from build123d import *

# Parameters (mm, degrees)
F1_DEPTH     = 10
F3_DEPTH     = 22
F4_DEPTH     = 48
F6_D         = 16
F6_DEPTH     = 54
F6_TIP       = 4.8068849522
F7_T1_DEPTH  = 14
F7_T4_ANGLE  = 180
F7_T5_DEPTH  = 46
F7_T7_DEPTH  = 29
F7_T10_ANGLE = 90
F7_T12_ANGLE = 90
F7_T13_DEPTH = 19.5
F7_T15_DEPTH = 19.5
F7_T17_DEPTH = 72.7186358508
F7_T19_DEPTH = 72.7186358508
F7_T22_ANGLE = 121.5042667192
F7_T26_DEPTH = 20.5
F7_S27_R     = 16.5
F7_T28_DEPTH = 12
F7_T32_DEPTH = 20.5
F7_S33_R     = 16.5
F7_T34_DEPTH = 12
F7_T36_ANGLE = 121.5042667192
F7_T38_ANGLE = 116.9914665616
F7_T40_ANGLE = 90
F7_T42_ANGLE = 90
F9_D         = 9


# Not quite as in the source:
# - a fillet or chamfer that OpenCascade refuses, or shapes differently, is made with other operations: its cross-section is extruded or revolved along the edge and cut away or added


with BuildPart() as f1:
    # F0 (on Top) → F1 (new body)
    with BuildSketch(Plane.XY):
        with BuildLine():
            ThreePointArc((11.9364175338, 7.315868811), (13.4742318051, 3.8006680023), (14, 0))
            ThreePointArc((14, 0), (-3.8006680023, -13.4742318051), (-11.9364175338, 7.315868811))
            Line((-11.9364175338, 7.315868811), (-49.9364175338, -54.684131189))
            ThreePointArc((-49.9364175338, -54.684131189), (-34.1993319977, -48.5257681949), (-24, -62))
            ThreePointArc((-24, -62), (-28.1005050634, -71.8994949366), (-38, -76))
            Line((-38, -76), (38, -76))
            ThreePointArc((38, -76), (25.7848012019, -55.1597574368), (49.9364175338, -54.684131189))
            Line((49.9364175338, -54.684131189), (11.9364175338, 7.315868811))
        make_face()
        with BuildLine():
            ThreePointArc((-24, -62), (-34.1993319977, -48.5257681949), (-49.9364175338, -54.684131189))
            ThreePointArc((-49.9364175338, -54.684131189), (-50.2151987981, -68.8402425632), (-38, -76))
            ThreePointArc((-38, -76), (-28.1005050634, -71.8994949366), (-24, -62))
        make_face()
        with BuildLine():
            ThreePointArc((-11.9364175338, 7.315868811), (-3.8006680023, -13.4742318051), (14, 0))
            ThreePointArc((14, 0), (13.4742318051, 3.8006680023), (11.9364175338, 7.315868811))
            ThreePointArc((11.9364175338, 7.315868811), (0, 14), (-11.9364175338, 7.315868811))
        make_face()
        with BuildLine():
            ThreePointArc((52, -62), (51.4742318051, -58.1993319977), (49.9364175338, -54.684131189))
            ThreePointArc((49.9364175338, -54.684131189), (25.7848012019, -55.1597574368), (38, -76))
            ThreePointArc((38, -76), (47.8994949366, -71.8994949366), (52, -62))
        make_face()
    extrude(amount=F1_DEPTH)

    # F2 (on face) → F3 (join)
    with BuildSketch(Plane.XZ.offset(76)):
        with BuildLine():
            ThreePointArc((8.7321245983, 10), (14.4279252818, 15.9946910076), (16.5, 24))
            ThreePointArc((16.5, 24), (0, 40.5), (-16.5, 24))
            ThreePointArc((-16.5, 24), (-14.4279252818, 15.9946910076), (-8.7321245983, 10))
            Line((-8.7321245983, 10), (8.7321245983, 10))
        make_face()
        with BuildLine():
            ThreePointArc((-8.7321245983, 10), (0, 7.5), (8.7321245983, 10))
            Line((8.7321245983, 10), (-8.7321245983, 10))
        make_face()
    extrude(amount=F3_DEPTH)

    # F2 (on face) → F4 (join)
    with BuildSketch(Plane.XZ.offset(76)):
        with BuildLine():
            Line((16.5, 10), (16.5, 24))
            ThreePointArc((16.5, 24), (14.4279252818, 15.9946910076), (8.7321245983, 10))
            Line((8.7321245983, 10), (16.5, 10))
        make_face()
        with BuildLine():
            ThreePointArc((8.7321245983, 10), (14.4279252818, 15.9946910076), (16.5, 24))
            ThreePointArc((16.5, 24), (0, 40.5), (-16.5, 24))
            ThreePointArc((-16.5, 24), (-14.4279252818, 15.9946910076), (-8.7321245983, 10))
            Line((-8.7321245983, 10), (8.7321245983, 10))
        make_face()
        with BuildLine():
            ThreePointArc((-8.7321245983, 10), (-14.4279252818, 15.9946910076), (-16.5, 24))
            Line((-16.5, 24), (-16.5, 10))
            Line((-16.5, 10), (-8.7321245983, 10))
        make_face()
    extrude(amount=-F4_DEPTH)

    # F6
    with Locations(Plane.XZ.offset(98)):
        with Locations((0, 24)):
            Hole(F6_D / 2, depth=F6_DEPTH)
            with Locations((0, 0, -(F6_DEPTH + F6_TIP / 2))):  # 118° drill point
                Cone(0, F6_D / 2, F6_TIP, mode=Mode.SUBTRACT)

    # F7: fillet of radius 2 on 15 edges, made by hand

    # F7_s2 → F7_t1 (cut)
    with BuildSketch(Plane.XY.offset(10)):
        with BuildLine():
            ThreePointArc((-16.5, -30), (-15.9142135624, -28.5857864376), (-14.5, -28))
            Line((-14.5, -28), (-16.5, -28))
            Line((-16.5, -28), (-16.5, -30))
        make_face()
        with BuildLine():
            ThreePointArc((16.5, -30), (15.9142135624, -28.5857864376), (14.5, -28))
            Line((14.5, -28), (16.5, -28))
            Line((16.5, -28), (16.5, -30))
        make_face()
    extrude(amount=F7_T1_DEPTH, mode=Mode.SUBTRACT)

    # F7_s3 → F7_t4 (revolve, cut)
    with BuildSketch(Plane.XY.offset(24)):
        with BuildLine():
            ThreePointArc((16.5, -30), (15.9142135624, -28.5857864376), (14.5, -28))
            Line((14.5, -28), (16.5, -28))
            Line((16.5, -28), (16.5, -30))
        make_face()
    revolve(axis=Axis((0, -28, 24), (0, -1, 0)), revolution_arc=F7_T4_ANGLE, mode=Mode.SUBTRACT)

    # F7_s6 → F7_t5 (join)
    with BuildSketch(Plane.XZ.offset(30)):
        with BuildLine():
            ThreePointArc((18.5, 10), (17.0857864376, 10.5857864376), (16.5, 12))
            Line((16.5, 12), (16.5, 10))
            Line((16.5, 10), (18.5, 10))
        make_face()
        with BuildLine():
            ThreePointArc((-18.5, 10), (-17.0857864376, 10.5857864376), (-16.5, 12))
            Line((-16.5, 12), (-16.5, 10))
            Line((-16.5, 10), (-18.5, 10))
        make_face()
    extrude(amount=F7_T5_DEPTH)

    # F7_s8 → F7_t7 (join)
    with BuildSketch(Plane.YZ.offset(-14.5)):
        with BuildLine():
            ThreePointArc((-26, 10), (-27.4142135624, 10.5857864376), (-28, 12))
            Line((-28, 12), (-28, 10))
            Line((-28, 10), (-26, 10))
        make_face()
    extrude(amount=F7_T7_DEPTH)

    # F7_s9 → F7_t10 (revolve)
    with BuildSketch(Plane.XZ.offset(30)):
        with BuildLine():
            ThreePointArc((-18.5, 10), (-17.0857864376, 10.5857864376), (-16.5, 12))
            Line((-16.5, 12), (-16.5, 10))
            Line((-16.5, 10), (-18.5, 10))
        make_face()
    revolve(axis=Axis((-14.5, -30, 10), (0, 0, -1)), revolution_arc=F7_T10_ANGLE)

    # F7_s11 → F7_t12 (revolve)
    with BuildSketch(Plane.XZ.offset(30)):
        with BuildLine():
            ThreePointArc((18.5, 10), (17.0857864376, 10.5857864376), (16.5, 12))
            Line((16.5, 12), (16.5, 10))
            Line((16.5, 10), (18.5, 10))
        make_face()
    revolve(axis=Axis((14.5, -30, 10), (0, 0, 1)), revolution_arc=F7_T12_ANGLE)

    # F7_s14 → F7_t13 (cut)
    with BuildSketch(Plane.YZ.offset(-38)):
        with BuildLine():
            ThreePointArc((-76, 8), (-75.4142135624, 9.4142135624), (-74, 10))
            Line((-74, 10), (-76, 10))
            Line((-76, 10), (-76, 8))
        make_face()
    extrude(amount=F7_T13_DEPTH, mode=Mode.SUBTRACT)

    # F7_s16 → F7_t15 (cut)
    with BuildSketch(Plane.YZ.offset(18.5)):
        with BuildLine():
            ThreePointArc((-76, 8), (-75.4142135624, 9.4142135624), (-74, 10))
            Line((-74, 10), (-76, 10))
            Line((-76, 10), (-76, 8))
        make_face()
    extrude(amount=F7_T15_DEPTH, mode=Mode.SUBTRACT)

    # F7_s18 → F7_t17 (cut)
    with BuildSketch(Plane(origin=(0, 0, 0), x_dir=(0, 0, 1), z_dir=(-0.5225620579, -0.8526012524, 0))):
        with BuildLine():
            ThreePointArc((10, 12), (9.4142135624, 13.4142135624), (8, 14))
            Line((8, 14), (10, 14))
            Line((10, 14), (10, 12))
        make_face()
    extrude(amount=F7_T17_DEPTH, mode=Mode.SUBTRACT)

    # F7_s20 → F7_t19 (cut)
    with BuildSketch(Plane(origin=(38, -62, 0), x_dir=(0, 0, 1), z_dir=(-0.5225620579, 0.8526012524, 0))):
        with BuildLine():
            ThreePointArc((10, 12), (9.4142135624, 13.4142135624), (8, 14))
            Line((8, 14), (10, 14))
            Line((10, 14), (10, 12))
        make_face()
    extrude(amount=F7_T19_DEPTH, mode=Mode.SUBTRACT)

    # F7_s21 → F7_t22 (revolve, cut)
    with BuildSketch(Plane.YZ.offset(38)):
        with BuildLine():
            ThreePointArc((-74, 10), (-75.4142135624, 9.4142135624), (-76, 8))
            Line((-76, 8), (-76, 10))
            Line((-76, 10), (-74, 10))
        make_face()
    revolve(axis=Axis((38, -62, 10), (0, 0, 1)), revolution_arc=F7_T22_ANGLE, mode=Mode.SUBTRACT)


with BuildPart() as f7_tool24:
    # F7_s25 → F7_t26 (new body)
    with BuildSketch(Plane.XY.offset(12)):
        with BuildLine():
            ThreePointArc((14.5, -76), (15.9142135624, -75.4142135624), (16.5, -74))
            Line((16.5, -74), (16.5, -76))
            Line((16.5, -76), (14.5, -76))
        make_face()
    extrude(amount=F7_T26_DEPTH)

    # F7_s27 → F7_t28 (cut, symmetric)
    with BuildSketch(Plane.XZ.offset(75)):
        with Locations((0, 24)):
            Circle(F7_S27_R)
    extrude(amount=F7_T28_DEPTH, both=True, mode=Mode.SUBTRACT)


with BuildPart() as f1_1:
    add(f1.part)

    # F7_t23: cut F7_tool24
    add(f7_tool24.part, mode=Mode.SUBTRACT)


with BuildPart() as f7_tool30:
    # F7_s31 → F7_t32 (new body)
    with BuildSketch(Plane.XY.offset(32.5)):
        with BuildLine():
            ThreePointArc((-14.5, -76), (-15.9142135624, -75.4142135624), (-16.5, -74))
            Line((-16.5, -74), (-16.5, -76))
            Line((-16.5, -76), (-14.5, -76))
        make_face()
    extrude(amount=-F7_T32_DEPTH)

    # F7_s33 → F7_t34 (cut, symmetric)
    with BuildSketch(Plane.XZ.offset(75)):
        with Locations((0, 24)):
            Circle(F7_S33_R)
    extrude(amount=F7_T34_DEPTH, both=True, mode=Mode.SUBTRACT)


with BuildPart() as f1_2:
    add(f1_1.part)

    # F7_t29: cut F7_tool30
    add(f7_tool30.part, mode=Mode.SUBTRACT)

    # F7_s35 → F7_t36 (revolve, cut)
    with BuildSketch(Plane(origin=(-38, -62, 0), x_dir=(0, 0, 1), z_dir=(0.5225620579, 0.8526012524, 0))):
        with BuildLine():
            ThreePointArc((8, -14), (9.4142135624, -13.4142135624), (10, -12))
            Line((10, -12), (10, -14))
            Line((10, -14), (8, -14))
        make_face()
    revolve(axis=Axis((-38, -62, 10), (0, 0, 1)), revolution_arc=F7_T36_ANGLE, mode=Mode.SUBTRACT)

    # F7_s37 → F7_t38 (revolve, cut)
    with BuildSketch(Plane(origin=(0, 0, 0), x_dir=(0, 0, 1), z_dir=(0.5225620579, -0.8526012524, 0))):
        with BuildLine():
            ThreePointArc((10, -12), (9.4142135624, -13.4142135624), (8, -14))
            Line((8, -14), (10, -14))
            Line((10, -14), (10, -12))
        make_face()
    revolve(axis=Axis((0, 0, 10), (0, 0, 1)), revolution_arc=F7_T38_ANGLE, mode=Mode.SUBTRACT)

    # F7_s39 → F7_t40 (revolve, cut)
    with BuildSketch(Plane.YZ.offset(18.5)):
        with BuildLine():
            ThreePointArc((-76, 8), (-75.4142135624, 9.4142135624), (-74, 10))
            Line((-74, 10), (-76, 10))
            Line((-76, 10), (-76, 8))
        make_face()
    revolve(axis=Axis((18.5, -76, 12), (0, 1, 0)), revolution_arc=F7_T40_ANGLE, mode=Mode.SUBTRACT)

    # F7_s41 → F7_t42 (revolve, cut)
    with BuildSketch(Plane.YZ.offset(-18.5)):
        with BuildLine():
            ThreePointArc((-76, 8), (-75.4142135624, 9.4142135624), (-74, 10))
            Line((-74, 10), (-76, 10))
            Line((-76, 10), (-76, 8))
        make_face()
    revolve(axis=Axis((-18.5, -76, 12), (0, -1, 0)), revolution_arc=F7_T42_ANGLE, mode=Mode.SUBTRACT)

    # F9 (through all)
    with Locations(Plane.XY.offset(10)):
        with Locations((38, -62), (0, 0), (-38, -62)):
            Hole(F9_D / 2)


solid = f1_2.part
Could you check a few things on this model? Use its own coordinates, in mm. A direction names the side the tool comes from. Coordinates: 2 decimals unless noted, no trailing zeros. Loops run counter-clockwise (first coordinate to the right, second up) from the corner with the lowest first, then second, coordinate; pieces in that order, holes last.
1. For P1, Ø10, axis at y = -25.5, z = 24.5, coming from the +X side; P2, Ø8, axis at x = 0, y = 0, coming from the -Z side; P3, Ø3.5, axis at y = -56.5, z = 18, coming from the -X side; P4, Ø5, axis at y = -54, z = 29, coming from the +X side, each with a flat end and sliding along its axis, tell me the tip position at first contact or that it passes through.
2. Imagine slicing it at A-A (z = 4). Please give me the cut outline in (x, y), and give its area (3 significant figures).
3. I need wall thicknesses on L1, parallel to Z at x = 0, y = -65.5; L2, parallel to Z at x = -15, y = -13; L3, parallel to Y at x = 0, z = 6. Which ranges of each line are inside material? Lowest first, please.
4. For faces 4 (the face through (-1, -21, 10)), 5 (the face through (1.041, -70.622, 31.932)), 6 (the face through (0, -28, 25)), 7 (the face through (-16.5, -52, 18)), which set-ups out of +Z, -Z, +X, -X, +Y, -Y let a thin tool reach every point of the face, with its end or its side?
5. We'd pull the mould along Y, two halves only. Please class faces 1 (the face through (0, 14, 4)), 2 (the face through (33.708, -60.648, 4.93)), 3 (the face through (-8, -98, 21)): released by +Y, released by -Y, zero draft, split by the parting line, or undercut.
Computed values:
1. P1: stops at x = 16.5
1. P2: passes through
1. P3: stops at x = -16.5
1. P4: stops at x = 16.31
2. outline: (-49.94, -54.68) arc R14 ccw to (-38, -76) - (38, -76) arc R14 ccw to (49.94, -54.68) - (11.94, 7.32) arc R14 ccw to (-11.94, 7.32) - close; hole circle Ø9 at (-38, -62); hole circle Ø9 at (0, 0); hole circle Ø9 at (38, -62)
2. area: 5,880 mm2
3. L1: z = 0 to 16, 32 to 40.5
3. L2: z = 0 to 10
3. L3: y = -76 to -4.5, 4.5 to 14
4. face 4: +Z, +Y
4. face 5: -Y
4. face 6: +Z, +X, -X, +Y
4. face 7: +Z, -X, +Y, -Y
5. face 1: released by +Y
5. face 2: undercut
5. face 3: released by -Y
